The model under review builds one solid part; all positions refer to its coordinate system, in mm. A direction names the side the tool comes from. Coordinates: 2 decimals unless noted, no trailing zeros. Order: outer loops, then holes, each group sorted by start corner. A loop starts at its lowest first (then second) coordinate and runs counter-clockwise, first axis right, second up. Notation, with made-up numbers: (56.25, 42.25) -> (70.25, 42.25) arc R20 cw to (70.25, 64.25) -> close; hole circle Ø7 at (15, -4). An arc over 180 degrees is marked (long way). Use one line per item in the form item = value. Start each with the question number.
(1) Take a section at C-C (z = 1.75). State the section outline as (x, y) points.
(2) Insertion check: pin 1 Ø1.5 at (y, z) = (9.5, 2) entering from +X; pin 2 Ø2.5 at (y, z) = (9.5, 3) entering from -X; pin 3 Ø5.5 at (x, z) = (31, 2) entering from +Y. Each pin has a flat end and moves straight along its axis. Give the tip position at first contact, or say it passes through.
(3) Take a section at A-A (x = 57.5). State the section outline as (y, z) points, then the cut area to 3 significant figures.
(4) Take a section at B-B (y = 12.5). State the section outline as (x, z) points.
(5) For faces 1 (the flat face through (118.872, 12, 3)), 2 (the flat face through (0, 12, 3)), 3 (the flat face through (59, 28.702, 8)), 4 (the flat face through (59, 0, 3)), 5 (the flat face through (59, 24.892, 3)), list the 3-axis set-ups (+Z, -Z, +X, -X, +Y, -Y) from which the entire face can be reached by the end or side of a thin tool; tool diameter is ignored.
(6) Wall thickness on line 1 along Y through (x, z) = (38.5, 2); line 2 along Z through (x, y) = (75, -2); line 3 along X through (y, z) = (9, 4.5): over which ranges is each line inside the solid? List them lowest first.
```python
from build123d import *

# Parameters (mm, degrees)
F0_W     = 118.872
F0_H     = 24.892
F1_DEPTH = 5.08
F2_W     = 126.492
F2_H     = 32.512
F2_W_2   = 118.872
F2_H_2   = 24.892
F3_DEPTH = 5.08


with BuildPart() as f1:
    # F0 (on Top) → F1 (new body)
    with BuildSketch(Plane.XY):
        with Locations((59.436, 12.446)):
            Rectangle(F0_W, F0_H)
    extrude(amount=F1_DEPTH)

    # F2 (on face) → F3 (join)
    with BuildSketch(Plane.XY.offset(5.08)):
        with Locations((59.436, 12.446)):
            Rectangle(F2_W, F2_H)
        with Locations((59.436, 12.446)):
            Rectangle(F2_W_2, F2_H_2, mode=Mode.SUBTRACT)
        with Locations((59.436, 12.446)):
            Rectangle(F2_W_2, F2_H_2)
    extrude(amount=F3_DEPTH)


solid = f1.part
```
Findings:
q1.outline = (0, 0) -> (118.87, 0) -> (118.87, 24.89) -> (0, 24.89) -> close
q2.pin_1 = 118.87
q2.pin_2 = 0
q2.pin_3 = 24.89
q3.outline = (-3.81, 5.08) -> (0, 5.08) -> (0, 0) -> (24.89, 0) -> (24.89, 5.08) -> (28.7, 5.08) -> (28.7, 10.16) -> (-3.81, 10.16) -> close
q3.area = 292 mm²
q4.outline = (-3.81, 5.08) -> (0, 5.08) -> (0, 0) -> (118.87, 0) -> (118.87, 5.08) -> (122.68, 5.08) -> (122.68, 10.16) -> (-3.81, 10.16) -> close
q5.face_1 = -Z, +X, +Y, -Y
q5.face_2 = -Z, -X, +Y, -Y
q5.face_3 = +Z, -Z, +X, -X, +Y
q5.face_4 = -Z, +X, -X, -Y
q5.face_5 = -Z, +X, -X, +Y
q6.line_1 = 0 to 24.89
q6.line_2 = 5.08 to 10.16
q6.line_3 = 0 to 118.87
